Autodesk Inventor part; units mm, degrees
ref_plane "YZ Plane" through (0, 0, 0) normal (1, 0, 0) x (0, 1, 0)
ref_plane "XZ Plane" through (0, 0, 0) normal (0, 1, 0) x (-1, 0, 0)
ref_plane "XY Plane" through (0, 0, 0) normal (0, 0, 1) x (1, 0, 0)
sketch "Sketch1" plane through (0, 0, 0) normal (0, 0, 1) x (1, 0, 0)
  circle A0 centre (0, 0) radius 5.5
  circle A1 centre (0, 0) radius 2.5
  dimension "d0" = 11
  dimension "d1" = 5
extrude "Extrusion1" add sketch "Sketch1" along normal blind 13.923
sketch "Sketch2" plane through (0, 0, 0) normal (0, 0, -1) x (-1, 0, 0)
  circle A0 centre (0, 0) radius 5.5
  circle A1 centre (0, 0) radius 11
  dimension "d4" = 22
extrude "Extrusion2" add sketch "Sketch2" against normal blind 3
sketch "Sketch3" plane through (0, 0, 0) normal (0, 0, -1) x (-1, 0, 0)
  line L0 (-6.245, 5) -> (-3, 5)
  circle A0 centre (0, 0) radius 1.5
  line L1 (-3, 5) -> (-3, -5)
  line L2 (-3, -5) -> (-6.245, -5)
  circle A1 centre (9.494, -1.674) radius 0.85
  spline S0 degree 3 poles (10.2296, -1.2481) (10.2738, -1.3244) (10.307, -1.4092) (10.3385, -1.5597) (10.3447, -1.6214) (10.3436, -1.712) (10.3419, -1.74) (10.3365, -1.7883) (10.3335, -1.8088) (10.3258, -1.8503) (10.3211, -1.8713) (10.3072, -1.9234) (10.2972, -1.9541) (10.2556, -2.0601) (10.2157, -2.1299) (10.1087, -2.269) (10.0384, -2.3333) (9.8581, -2.452) (9.7422, -2.496) (9.5082, -2.5317) (9.39, -2.526) (9.1776, -2.4693) (9.0836, -2.4258) (8.9226, -2.3102) (8.8553, -2.243) (8.7497, -2.0936) (8.7103, -2.0147) (8.6611, -1.8594) (8.648, -1.7853) (8.6432, -1.6739) (8.644, -1.6375) (8.6494, -1.5744) (8.653, -1.5477) (8.6628, -1.4942) (8.669, -1.4673) (8.6873, -1.4034) (8.7006, -1.3666) (8.7492, -1.2563) (8.7927, -1.1869) (8.912, -1.0459) (8.9921, -0.9805) (9.1784, -0.8769) (9.2836, -0.8435) (9.5106, -0.8156) (9.6296, -0.8269) (9.8522, -0.8944) (9.955, -0.9506) (10.1164, -1.0872) (10.1799, -1.1623) (10.2296, -1.2481) knots -0.565469 -0.565469 -0.565469 -0.565469 -0.536596 -0.536596 -0.517611 -0.517611 -0.509175 -0.509175 -0.50297 -0.50297 -0.496493 -0.496493 -0.486731 -0.486731 -0.461904 -0.461904 -0.431221 -0.431221 -0.390112 -0.390112 -0.351113 -0.351113 -0.31806 -0.31806 -0.288721 -0.288721 -0.262067 -0.262067 -0.23952 -0.23952 -0.228596 -0.228596 -0.220512 -0.220512 -0.212256 -0.212256 -0.200543 -0.200543 -0.176006 -0.176006 -0.144684 -0.144684 -0.110272 -0.110272 -0.071492 -0.071492 -0.032498 -0.032498 0 0 0 0
  circle A2 centre (9.494, -1.674) radius 1.35
  arc A3 (0, -8) -> (-6.245, 5) centre (0, 0) ccw
  arc A4 (-6.245, -5) -> (0, -8) centre (0, 0) ccw
  circle A5 centre (-4.074, -8.737) radius 0.85
  spline S1 degree 3 poles (-3.2275, -8.6604) (-3.2176, -8.7695) (-3.229, -8.877) (-3.2876, -9.0751) (-3.3329, -9.1647) (-3.4588, -9.3344) (-3.5435, -9.4107) (-3.7198, -9.5152) (-3.8078, -9.5499) (-3.9747, -9.5845) (-4.0515, -9.5903) (-4.1887, -9.5813) (-4.248, -9.5712) (-4.333, -9.547) (-4.3592, -9.5382) (-4.4041, -9.5206) (-4.4229, -9.5123) (-4.4611, -9.4941) (-4.4802, -9.484) (-4.5275, -9.4567) (-4.5549, -9.4386) (-4.6492, -9.3685) (-4.7078, -9.3092) (-4.8155, -9.1642) (-4.8589, -9.0767) (-4.9231, -8.8674) (-4.9328, -8.7429) (-4.9006, -8.5082) (-4.8622, -8.3976) (-4.7491, -8.2109) (-4.6814, -8.1333) (-4.5263, -8.0114) (-4.4435, -7.9656) (-4.2507, -7.8985) (-4.1412, -7.8825) (-3.9721, -7.8911) (-3.9136, -7.9002) (-3.8251, -7.9236) (-3.7941, -7.9337) (-3.7394, -7.9552) (-3.7153, -7.9659) (-3.6658, -7.9908) (-3.6405, -8.0053) (-3.5776, -8.0455) (-3.5413, -8.0731) (-3.4268, -8.1755) (-3.361, -8.262) (-3.2655, -8.4537) (-3.2369, -8.5564) (-3.2275, -8.6604) knots -0.566086 -0.566086 -0.566086 -0.566086 -0.531825 -0.531825 -0.498779 -0.498779 -0.460694 -0.460694 -0.429612 -0.429612 -0.405256 -0.405256 -0.386838 -0.386838 -0.378505 -0.378505 -0.372312 -0.372312 -0.365791 -0.365791 -0.355852 -0.355852 -0.330056 -0.330056 -0.298514 -0.298514 -0.25701 -0.25701 -0.218398 -0.218398 -0.185587 -0.185587 -0.156394 -0.156394 -0.123104 -0.123104 -0.105349 -0.105349 -0.095573 -0.095573 -0.087672 -0.087672 -0.078924 -0.078924 -0.065227 -0.065227 -0.032657 -0.032657 0 0 0 0
  circle A6 centre (-4.074, -8.737) radius 1.35
  circle A7 centre (-4.82, 8.349) radius 0.85
  spline S2 degree 3 poles (-4.1123, 8.8197) (-4.052, 8.7291) (-4.0084, 8.6259) (-3.9677, 8.4209) (-3.9647, 8.3234) (-3.9919, 8.1375) (-4.0188, 8.0509) (-4.0994, 7.8893) (-4.1522, 7.8154) (-4.2455, 7.7212) (-4.2773, 7.6934) (-4.3337, 7.6513) (-4.3572, 7.6355) (-4.4041, 7.6072) (-4.4275, 7.5946) (-4.4822, 7.5683) (-4.5139, 7.5553) (-4.6086, 7.5231) (-4.6731, 7.5092) (-4.8426, 7.4929) (-4.947, 7.5022) (-5.1521, 7.5589) (-5.2492, 7.6077) (-5.4281, 7.7434) (-5.5042, 7.8321) (-5.6193, 8.0357) (-5.6549, 8.1509) (-5.6758, 8.3693) (-5.6674, 8.4725) (-5.6185, 8.6517) (-5.5851, 8.7291) (-5.4963, 8.8702) (-5.4427, 8.9337) (-5.3552, 9.0101) (-5.3302, 9.0296) (-5.2865, 9.0599) (-5.2685, 9.0714) (-5.2323, 9.0926) (-5.2143, 9.1023) (-5.1705, 9.1239) (-5.1446, 9.1351) (-5.0727, 9.162) (-5.0263, 9.175) (-4.8823, 9.2025) (-4.7852, 9.2034) (-4.5796, 9.1723) (-4.4735, 9.1329) (-4.2735, 9.0117) (-4.182, 8.9246) (-4.1123, 8.8197) knots -0.567177 -0.567177 -0.567177 -0.567177 -0.53086 -0.53086 -0.500336 -0.500336 -0.472721 -0.472721 -0.445441 -0.445441 -0.432747 -0.432747 -0.42424 -0.42424 -0.416254 -0.416254 -0.405955 -0.405955 -0.386117 -0.386117 -0.354442 -0.354442 -0.320748 -0.320748 -0.283148 -0.283148 -0.243084 -0.243084 -0.208567 -0.208567 -0.181377 -0.181377 -0.155642 -0.155642 -0.146036 -0.146036 -0.139581 -0.139581 -0.133402 -0.133402 -0.124853 -0.124853 -0.110096 -0.110096 -0.079394 -0.079394 -0.04201 -0.04201 0 0 0 0
  circle A8 centre (-4.82, 8.349) radius 1.35
  circle A9 centre (0, 0) radius 1.5
  circle A10 centre (0, 0) radius 8
  dimension "d7" = 2.7
  dimension "d8" = 2.7
  dimension "d9" = 2.7
extrude "Extrusion3" add sketch "Sketch3" along normal blind 3 contours A1 | A2 | A5 | A6 | A7 | A8
sketch "Sketch4" plane through (0, 0, 13.923) normal (0, 0, 1) x (1, 0, 0)
  circle A0 centre (0, 0) radius 2.5
  line L0 (-7.7, 0) -> (7.7, 0)
  point P0 (4, 0)
  dimension "d12" = 4
hole "Hole1" at (4, 0, 13.923) direction (0, 0, -1) diameter 1.694 depth 3
pattern_circular "Circular Pattern1" count 3 over 360 about axis through (0, 0, -10) along (0, 0, 1) of "Hole1"
sketch "Sketch5" plane through (4.074, -8.737, -3) normal (0, 0, -1) x (-1, 0, 0)
  circle A0 centre (0, 0) radius 1.35
  point P0 (4.074, 8.737)
hole "Hole2" at (4.074, -8.737, -3) direction (0, 0, 1) diameter 1.694 depth 3 tip angle 118
properties part number "ss_inner_guide_bottom"
The model under review builds one solid part; all positions refer to its coordinate system, in mm. A direction names the side the tool comes from. Give positions to 0.01 mm unless a question says otherwise; leave off trailing zeros. Write each loop counter-clockwise with the first axis right and the second up, starting at its lowest first coordinate (ties: lowest second). Pieces come first, ordered by that corner, then holes. Notation, with made-up numbers: M 7,68.5 L 18,68.5 A19 cw 18,88.5 Z; hole C 32,43.5 d2. An arc over 180 degrees is marked long. Write item = value, one per line. Start each with the question number.
Q1. We need section B-B (x = 0). State the section outline as (y, z) points.
Q2. We need section D-D (y = -4.75). State the section outline as (x, z) points.
Q3. Machinability: for faces 4 (the face through (3.234, -8.847, -1.479)), 5 (the face through (-9, -2, -3)), 6 (the face through (-2, -3, 10.923)), which of the approach directions +Z, -Z, +X, -X, +Y, -Y give a long, thin tool a straight path to every point of the face, cutting with its end or side? Answer none if there is none.
Q4. Clearance check with flat-ended pins moving along their axes: pin 1 (1.5 mm diameter, centred on x = -3.5, y = -7, fed in from +Z); pin 2 (1.4 mm diameter, centred on x = -2, y = 3.46, fed in from -Z); pin 3 (0.8 mm diameter, centred on x = 4, y = 0, fed in from +Z). State where each tip first meets the part, or that it passes through.
Q5. Mouldability with a two-part tool opening along X and no side actions: class faces 1 (the face through (-2, 3, 10.923)), 2 (the face through (-8.145, -1.733, -1.479)), 3 (the face through (5, 8, -3)) as released by +X, released by -X, zero draft, split by the parting line, or undercut.
Q6. For line 1 (Z direction, x = 1.25, y = -4.75); line 2 (Z direction, x = 2.75, y = -6.25); line 3 (Y direction, x = 0, z = 4.5), list the stretches that pass through material, from the lowest coordinate up.
Q7. We need section A-A (y = 0). State the section outline as (x, z) points, plus the area to 3 significant figures.
Q8. We need section C-C (z = 9.25). State the section outline as (x, y) points, plus the area to 3 significant figures.
Result set:
q1.outline = M -11,0 L -2.5,0 L -2.5,13.92 L -5.5,13.92 L -5.5,3 L -11,3 Z; M 2.5,0 L 11,0 L 11,3 L 5.5,3 L 5.5,13.92 L 2.5,13.92 Z
q2.outline = M -9.92,0 L 9.92,0 L 9.92,3 L 2.77,3 L 2.77,13.92 L -2.77,13.92 L -2.77,3 L -9.92,3 Z
q3.face_4 = -Z
q3.face_5 = -Z, +X, -X, +Y, -Y
q3.face_6 = +Z
q4.pin_1 = 3
q4.pin_2 = 0
q4.pin_3 = 10.92
q5.face_1 = undercut
q5.face_2 = split by the parting line
q5.face_3 = zero draft
q6.line_1 = 0 to 13.92
q6.line_2 = 0 to 3
q6.line_3 = -5.5 to -2.5, 2.5 to 5.5
q7.outline = M -11,0 L -2.5,0 L -2.5,13.92 L -5.5,13.92 L -5.5,3 L -11,3 Z; M 2.5,0 L 11,0 L 11,3 L 5.5,3 L 5.5,13.92 L 4.85,13.92 L 4.85,10.92 L 3.15,10.92 L 3.15,13.92 L 2.5,13.92 Z
q7.area = 111 mm2
q8.outline = C 0,0 d11; hole C 0,0 d5
q8.area = 75.4 mm2
